Drawing for the job (mm, zero at the part's lowest x, y, z). Round coordinates to 2 decimals unless told otherwise and drop trailing zeros. Loops run counter-clockwise (first coordinate to the right, second up) from the corner with the lowest first, then second, coordinate; pieces in that order, holes last. Notation, with made-up numbers: (-0.75, 81.5) - (20.25, 81.5) arc R23 ccw to (20.25, 119.5) - close; hole circle Ø7 at (35, -11). An arc over 180 degrees is marked (long way). Put each result on its own line as item: value.
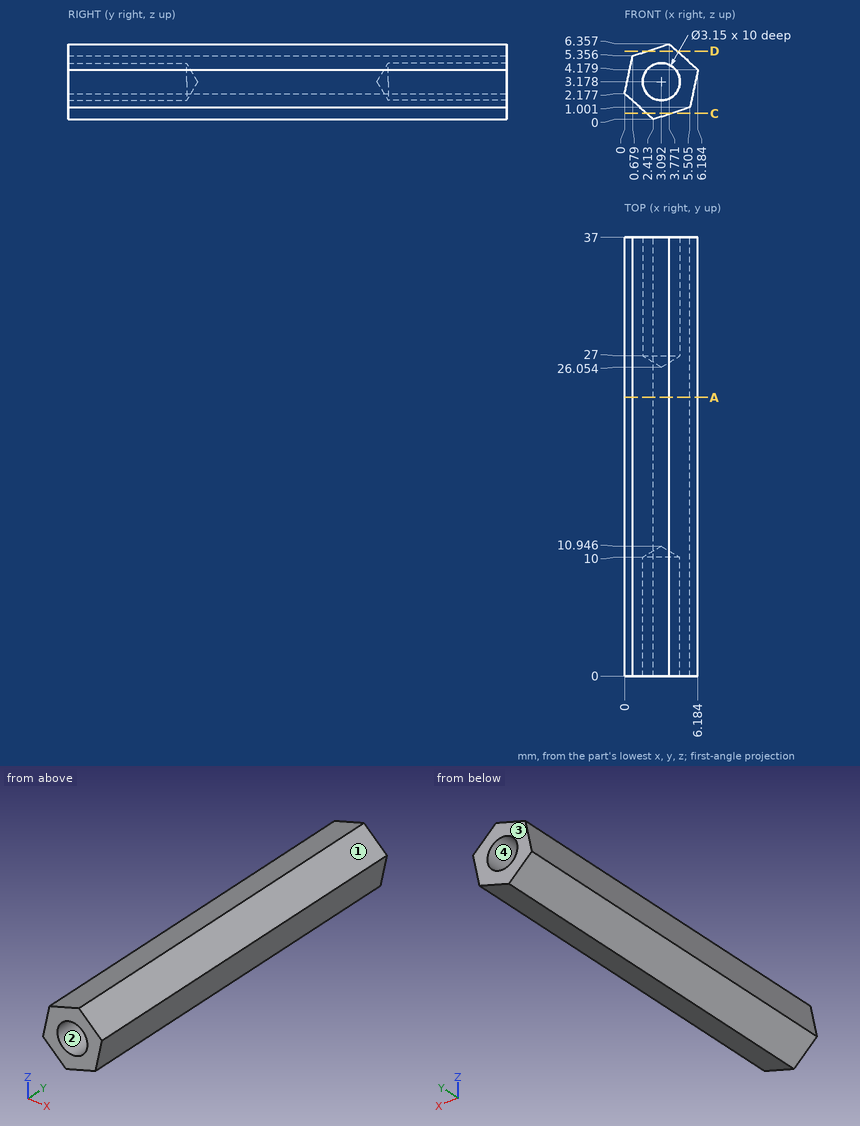
1. Band-saw the part on D-D (z = 5.75). List the corners of the cut face in (x, y).
A:
outline: (1.9, 0) - (4.44, 0) - (4.44, 37) - (1.9, 37) - close
2. Pin check, flat tips, straight feed: P1, Ø3.5, axis at x = 3.09, z = 3.18, coming from the +Y side; P2, Ø1.5, axis at y = 21, z = 1, coming from the -X side (1 decimal). Stop position of each tip, or through.
A:
P1: stops at y = 37
P2: stops at x = 0.5
3. Two-plate mould, pull along X, no slides. Class the marked faces 1, 2, 3 and 4: pulls with the +X half, pulls with the -X half, needs draft (parallel to the pull), parting line crosses it, or undercut.
A:
face 1: pulls with the +X half
face 2: undercut
face 3: needs draft
face 4: undercut
4. Band-saw the part on C-C (z = 0.5). List the corners of the cut face in (x, y).
A:
outline: (1.86, 0) - (3.96, 0) - (3.96, 37) - (1.86, 37) - close
5. Band-saw the part on A-A (y = 23.5). List the corners of the cut face in (x, z) (1 decimal).
A:
outline: (0, 2.2) - (2.4, 0) - (5.5, 1) - (6.2, 4.2) - (3.8, 6.4) - (0.7, 5.4) - close
6. Probe line 1 along X through (y, z) = (31.5, 3.75) (1 decimal); line 2 along Z through (x, y) = (3.75, 9.5); line 3 along Z through (x, y) = (4.25, 30.5) (1 decimal). List the from-to ranges inside material, lowest first. Write a range as [from, to].
A:
line 1: x = [0.3, 1.6], [4.6, 6.1]
line 2: z = [0.43, 1.75], [4.61, 6.35]
line 3: z = [0.6, 2.1], [4.2, 5.9]
